Geometry check sheet. Reference: the model listing, model coordinates, mm. A direction names the side the tool comes from. Round coordinates to 2 decimals unless told otherwise and drop trailing zeros. Write each loop counter-clockwise with the first axis right and the second up, starting at its lowest first coordinate (ties: lowest second). Pieces come first, ordered by that corner, then holes. Notation, with made-up numbers: M 27.25,-7 L 31.25,-7 A26 ccw 31.25,13 Z; hole C -15,65.5 d10. An arc over 180 degrees is marked long. Use a Markdown table: item, result.
Autodesk Inventor part; units mm, degrees
ref_plane "Work Plane2" through (0, 19.05, 0) normal (0, 1, 0) x (1, 0, 0)
ref_plane "Work Plane1" through (0, 19.05, 0) normal (0, 1, 0) x (1, 0, 0)
ref_plane "YZ Plane" through (0, 0, 0) normal (1, 0, 0) x (0, 1, 0)
sketch "Sketch1" plane through (0, 0, 0) normal (0, 1, 0) x (-1, 0, 0)
  circle A0 centre (0, 0) radius 8.0645
  circle A1 centre (0, -44.45) radius 6.985
  circle A2 centre (0, 44.45) radius 6.985
  line L0 (-39.6048, 88.9) -> (39.6048, 88.9)
  line L1 (39.6048, 88.9) -> (39.6048, -88.9)
  line L2 (39.6048, -88.9) -> (-39.6048, -88.9)
  line L3 (-39.6048, -88.9) -> (-39.6048, 88.9)
  line L4 (-39.6048, 88.9) -> (39.6048, -88.9) construction
  line L5 (39.6048, 88.9) -> (-39.6048, -88.9) construction
  line L6 (10.9754, 63.5) -> (10.9754, 0) construction
  point P0 (0, 0)
  point P1 (0, 0)
  dimension "d0" = 16.129
  dimension "d1" = 13.97
  dimension "d2" = 13.97
  dimension "d28" = 177.8
  dimension "d82" = 44.45
  dimension "d83" = 44.45
extrude "Extrusion4" add sketch "Sketch1" along normal blind 19.05
ref_plane "Work Plane2" through (0, 19.05, 0) normal (0, 1, 0) x (1, 0, 0)
sketch "Sketch2" plane through (0, 19.05, 0) normal (0, 1, 0) x (1, 0, 0)
  circle A0 centre (-11.2395, 0) radius 1.25
  circle A1 centre (0, 0) radius 7.94
  circle A2 centre (5.6197, -9.7337) radius 1.25
  circle A3 centre (5.6198, 9.7337) radius 1.25
  dimension "d11" = 2.5
  dimension "d12" = 11.2395
  dimension "d15" = 360
ref_plane "Work Plane1" through (0, 19.05, 0) normal (0, 1, 0) x (1, 0, 0)
extrude "Extrusion5" cut sketch "Sketch2" against normal up to next contours A0 | A2 | A3
sketch "Sketch6" plane through (0, 19.05, 0) normal (0, 1, 0) x (1, 0, 0)
  circle A0 centre (0, 0) radius 8.0645
  arc A1 (0, 18.8395) -> (0, -18.8395) centre (0, 0) ccw
  circle A2 centre (-11.2395, 0) radius 1.25
  circle A3 centre (0, -44.45) radius 6.985
  circle A4 centre (0, -44.45) radius 6.985
  arc A5 (0, -31.75) -> (0, -57.15) centre (0, -44.45) ccw
  line L0 (54.9709, 0) -> (-46.1054, 0) construction
  arc A6 (0, 57.15) -> (0, 31.75) centre (0, 44.45) ccw
  line L1 (10.0601, -57.15) -> (10.0601, -88.9)
  line L2 (10.0601, -88.9) -> (-39.6048, -88.9)
  line L3 (-39.6048, 88.9) -> (-39.6048, -88.9)
  line L4 (-39.6048, -88.9) -> (-39.6048, 88.9)
  line L5 (-39.6048, 88.9) -> (10.0601, 88.9)
  line L6 (10.0601, 57.15) -> (10.0601, 88.9)
  line L7 (0, 57.15) -> (10.0601, 57.15)
  line L8 (0, 31.75) -> (0, 18.8395)
  line L9 (0, -18.8395) -> (0, -31.75)
  line L10 (10.0601, -57.15) -> (0, -57.15)
  point P0 (0, 0)
  dimension "d77" = 6.35
  dimension "d103" = 12.7
sketch "Sketch12" plane through (0, 19.05, 0) normal (0, 1, 0) x (1, 0, 0)
  line L0 (39.6048, -88.9) -> (39.6048, 88.9)
  line L1 (39.6048, -82.55) -> (19.685, -82.55)
  line L2 (19.685, -82.55) -> (19.685, 82.55)
  line L3 (19.685, 82.55) -> (39.6048, 82.55)
  line L4 (39.6048, 82.55) -> (39.6048, -82.55)
  line L5 (39.6048, 88.9) -> (-39.6048, 88.9)
  line L6 (-39.6048, -88.9) -> (39.6048, -88.9)
  circle A0 centre (0, -44.45) radius 6.985
  point P0 (0, 0)
  point P1 (12.7, 88.9)
  point P2 (12.7, -88.9)
  point P3 (0, 88.9)
  point P4 (10.0601, 88.9)
  point P5 (10.0601, -88.9)
  dimension "d72" = 6.35
  dimension "d73" = 6.35
  dimension "d74" = 12.7
extrude "Extrusion10" cut sketch "Sketch12" against normal up to next contours L1 L2 L3 L0
sketch "Sketch13" plane through (39.6048, 0, 88.9) normal (1, 0, 0) x (0, 0, -1)
  line L0 (0, 0) -> (0, 19.05)
  line L1 (171.45, 0) -> (6.35, 0)
  line L2 (0, 19.05) -> (6.35, 19.05)
  line L3 (6.35, 19.05) -> (6.35, 0)
  line L4 (6.35, 0) -> (0, 0)
  line L5 (0, 0) -> (0, 19.05)
  line L6 (171.45, 19.05) -> (171.45, 0)
  line L7 (177.8, 19.05) -> (177.8, 0)
  line L8 (171.45, 19.05) -> (177.8, 19.05)
  line L9 (177.8, 19.05) -> (177.8, 0)
  line L10 (177.8, 0) -> (171.45, 0)
  line L11 (171.45, 0) -> (171.45, 19.05)
  point P0 (88.9, 0)
extrude "Extrusion11" add sketch "Sketch13" along normal blind 50.8
sketch "Sketch14" plane through (19.685, 19.05, 82.55) normal (1, 0, 0) x (0, 0, -1)
  line L0 (0, 0) -> (0, -19.05)
  line L1 (165.1, -19.05) -> (0, -19.05)
  line L2 (0, 0) -> (165.1, 0)
  line L3 (165.1, 0) -> (165.1, -19.05)
  line L4 (165.1, -19.05) -> (0, -19.05)
  line L5 (0, -19.05) -> (0, 0)
  point P0 (82.55, -19.05)
extrude "Extrusion12" add sketch "Sketch14" along normal blind 12.7
extrude "Extrusion14" cut sketch "Sketch6" against normal up to next contours A1 L9 A5 L10 L1 L2 L3 L5 L6 L7 A6 L8
sketch "Sketch16" plane through (0, 19.05, -31.75) normal (-1, 0, 0) x (0, 0, 1)
  line L0 (-15.875, -3.048) -> (-15.875, -16.002)
  line L1 (-19.685, -16.002) -> (-19.685, -3.048)
  line L2 (-19.685, -3.048) -> (-15.875, -3.048)
  line L3 (-9.525, -3.048) -> (-5.715, -3.048)
  line L4 (-19.685, -16.002) -> (-15.875, -16.002)
  line L5 (-9.525, -16.002) -> (-5.715, -16.002)
  line L6 (-5.715, -3.048) -> (-5.715, -16.002)
  line L7 (-9.525, -3.048) -> (-9.525, -16.002)
  point P0 (31.75, -19.05)
  dimension "d106" = 3.81
  dimension "d112" = 3.81
extrude "Extrusion15" cut sketch "Sketch16" along normal up to next
mirror "Mirror3" about plane through (0, 0, 0) normal (0, 0, 1) of "Extrusion15"
fillet "Fillet8" radius 12.7 4 edges at (10.0601, 9.525, 57.15) (10.0601, 9.525, 88.9) (10.0601, 9.525, -88.9) (10.0601, 9.525, -57.15)
properties part number "AlteredPlatform"
Item 1: Access from +Z, -Z, +X, -X, +Y, -Y to the whole of each face (thin tool, end or side, straight path). Record for faces 1 (the face through (-7, 3.048, 50)), 2 (the face through (0, 10, -25)), 3 (the face through (32.385, 10, 1)).
Outcome:
| item | result |
|---|---|
| face 1 | -X |
| face 2 | -X, +Y, -Y |
| face 3 | +X, +Y, -Y |
Item 2: Cross-section at A-A, the plane z = 44.45. Record the cut outline in (x, y) (3 decimals), and give its area (3 significant figures).
Outcome:
| item | result |
|---|---|
| outline | M -12.7,0 L -6.985,0 L -6.985,19.05 L -12.7,19.05 Z; M 6.985,0 L 32.385,0 L 32.385,19.05 L 6.985,19.05 Z |
| area | 593 mm2 |
Item 3: Cross-section at B-B, the plane x = 67. Record the cut outline in (y, z).
Outcome:
| item | result |
|---|---|
| outline | M 0,-88.9 L 19.05,-88.9 L 19.05,-82.55 L 0,-82.55 Z; M 0,82.55 L 19.05,82.55 L 19.05,88.9 L 0,88.9 Z |
Item 4: Cross-section at C-C, the plane z = 21. Record the cut outline in (x, y) (3 decimals).
Outcome:
| item | result |
|---|---|
| outline | M 0,0 L 32.385,0 L 32.385,19.05 L 0,19.05 Z |
Item 5: Go/stop test with flat-tipped pins: pin 1 (10.5 mm diameter, centred on y = 13, z = 25.5, fed in from -X); pin 2 (2 mm diameter, centred on x = 5.62, z = 9.73, fed in from +Y); pin 3 (5 mm diameter, centred on x = -9.5, y = 9, fed in from -Z); pin 4 (1 mm diameter, centred on y = 6.5, z = -51.5, fed in from -X). Record where each tip stops, or that it passes through.
Outcome:
| item | result |
|---|---|
| pin 1 | stops at x = 0 |
| pin 2 | passes through |
| pin 3 | stops at z = -55.05 |
| pin 4 | stops at x = -10.61 |
Item 6: Mould release check, pull along Z, two halves, no side actions. Record for faces 4 (the face through (13.9, 9.4, 85.3)), 5 (the face through (10.06, 10, 73)), 6 (the face through (-5, 10, -37.465)), 7 (the face through (56, 9, -88.9)): +Z half, -Z half, draft (parallel to the pull), parting line (faces both ways), or undercut.
Outcome:
| item | result |
|---|---|
| face 4 | +Z half |
| face 5 | draft |
| face 6 | undercut |
| face 7 | -Z half |
Item 7: Cross-section at D-D, the plane y = 7.75. Count the separate pieces of the cut face and the enclosed holes in it, and give its area (3 significant figures).
Outcome:
| item | result |
|---|---|
| separate pieces | 3 |
| enclosed holes | 4 |
| area | 6,280 mm2 |
Item 8: Material ranges on line 1 along Z through (x, y) = (84, 10.5); line 2 along Z through (x, y) = (2.5, 16.5); line 3 along X through (y, z) = (12.75, -10.5) (3 decimals), recorded low to high. Write a range as from..to.
Outcome:
| item | result |
|---|---|
| line 1 | z = -88.9..-82.55, 82.55..88.9 |
| line 2 | z = -58.1..-50.97, -37.93..-7.67, 7.67..37.93, 50.97..58.1 |
| line 3 | x = -15.642..4.632, 6.607..32.385 |
